Part model, mm, in its own coordinate system. Coordinates: 2 decimals unless noted, no trailing zeros. Write each loop counter-clockwise with the first axis right and the second up, starting at its lowest first coordinate (ties: lowest second). Pieces come first, ordered by that corner, then holes. Notation, with made-up numbers: (51, -5) -> (89, -5) arc R8 cw to (89, -1) -> close; hole circle Ø2 at (79.25, 62.5). An arc over 180 degrees is marked (long way). One line per question, with ' | ' between items. Start each with the question number.
Item 1: Saw through at B-B (x = 228.6). List the corners of the cut face in (y, z) (3 decimals), and give its area (3 significant figures).
Item 2: Probe probe 1 along Z at (x, y) = (228.6, 2); probe 2 along X at (y, z) = (0.7, -63.5); probe 3 along Z at (x, y) = (187, 1.05). List the from-to ranges inside material, lowest first. Write a range as [from, to].
Item 3: Saw through at C-C (z = -8.5). List the corners of the cut face in (x, y) (3 decimals).
Item 4: Pin check, flat tips, straight feed: pin 1 (1 mm diameter, centred on y = 1.5, z = -8, fed in from -X); pin 2 (1.6 mm diameter, centred on y = 1, z = -120.5, fed in from +X); pin 3 (1 mm diameter, centred on x = 63.5, y = 2, fed in from +Z). Stop position of each tip, or through.
Item 5: Saw through at D-D (x = 60.5). List the corners of the cut face in (y, z) (3 decimals).
Item 6: Saw through at A-A (z = -63.5). List the corners of the cut face in (x, y) (3 decimals), and give its area (3 significant figures).
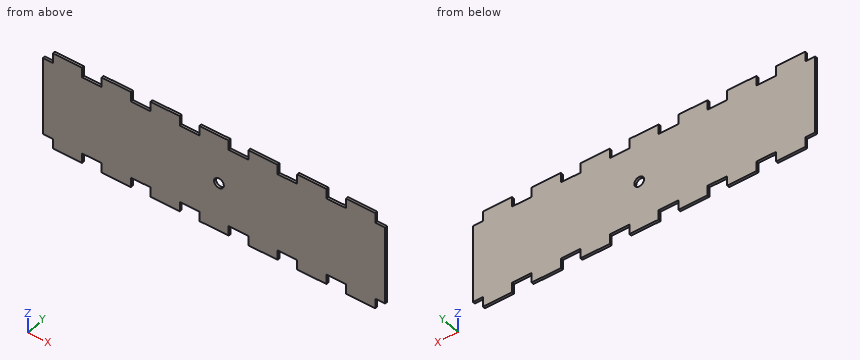
Autodesk Inventor part; units mm, degrees
ref_plane "YZ Plane" through (0, 0, 0) normal (1, 0, 0) x (0, 1, 0)
ref_plane "XZ Plane" through (0, 0, 0) normal (0, 1, 0) x (-1, 0, 0)
ref_plane "XY Plane" through (0, 0, 0) normal (0, 0, 1) x (1, 0, 0)
sketch "Sketch1" plane through (0, 0, 0) normal (0, 1, 0) x (-1, 0, 0)
  line L0 (0, 0) -> (-444.5, 0)
  line L1 (-444.5, 0) -> (-444.5, -127)
  line L2 (-444.5, -127) -> (0, -127)
  line L3 (0, -127) -> (0, 0)
  dimension "d0" = 444.5
  dimension "d1" = 127
extrude "Extrusion1" add sketch "Sketch1" along normal blind 3.175
sketch "Sketch2" plane through (0, 3.175, 0) normal (0, 1, 0) x (1, 0, 0)
  line L0 (0, 127) -> (0, 0)
  line L1 (0, 114.3) -> (12.7, 114.3)
  line L2 (12.7, 114.3) -> (12.7, 127)
  line L3 (444.5, 127) -> (0, 127)
  line L4 (50.8, 127) -> (50.8, 114.3)
  line L5 (50.8, 114.3) -> (76.2, 114.3)
  line L6 (76.2, 114.3) -> (76.2, 127)
  line L7 (114.3, 127) -> (114.3, 114.3)
  line L8 (114.3, 114.3) -> (139.7, 114.3)
  line L9 (139.7, 114.3) -> (139.7, 127)
  line L10 (177.8, 127) -> (177.8, 114.3)
  line L11 (177.8, 114.3) -> (203.2, 114.3)
  line L12 (203.2, 114.3) -> (203.2, 127)
  line L13 (241.3, 127) -> (241.3, 114.3)
  line L14 (241.3, 114.3) -> (266.7, 114.3)
  line L15 (266.7, 114.3) -> (266.7, 127)
  line L16 (304.8, 127) -> (304.8, 114.3)
  line L17 (304.8, 114.3) -> (330.2, 114.3)
  line L18 (330.2, 114.3) -> (330.2, 127)
  line L19 (368.3, 127) -> (368.3, 114.3)
  line L20 (368.3, 114.3) -> (393.7, 114.3)
  line L21 (393.7, 114.3) -> (393.7, 127)
  line L22 (431.8, 127) -> (431.8, 114.3)
  line L23 (431.8, 114.3) -> (444.5, 114.3)
  line L24 (444.5, 0) -> (444.5, 127)
  line L25 (0, 114.3) -> (0, 127)
  line L26 (50.8, 127) -> (76.2, 127)
  line L27 (114.3, 127) -> (139.7, 127)
  line L28 (177.8, 127) -> (203.2, 127)
  line L29 (241.3, 127) -> (266.7, 127)
  line L30 (304.8, 127) -> (330.2, 127)
  line L31 (368.3, 127) -> (393.7, 127)
  line L32 (431.8, 127) -> (444.5, 127)
  line L33 (0, 127) -> (12.7, 127)
  point P0 (444.5, 114.3)
  point P1 (12.7, 127)
  dimension "d4" = 12.7
  dimension "d6" = 12.7
  dimension "d7" = 12.7
  dimension "d8" = 12.7
  dimension "d9" = 25.4
  dimension "d10" = 38.1
  dimension "d11" = 25.4
  dimension "d12" = 38.1
  dimension "d13" = 25.4
  dimension "d14" = 38.1
  dimension "d15" = 25.4
  dimension "d16" = 38.1
  dimension "d17" = 25.4
  dimension "d18" = 38.1
  dimension "d19" = 25.4
  dimension "d20" = 38.1
  dimension "d22" = 0
  dimension "d42" = 12.7
  dimension "d53" = 38.1
extrude "Extrusion2" cut sketch "Sketch2" against normal through all
sketch "Sketch3" plane through (0, 3.175, 0) normal (0, 1, 0) x (1, 0, 0)
  line L0 (0, 0) -> (444.5, 0)
  line L1 (0, 0) -> (12.7, 0)
  line L2 (12.7, 0) -> (12.7, 12.7)
  line L3 (12.7, 12.7) -> (0, 12.7)
  line L4 (0, 12.7) -> (0, 0)
  line L5 (50.8, 0) -> (76.2, 0)
  line L6 (76.2, 0) -> (76.2, 12.7)
  line L7 (76.2, 12.7) -> (50.8, 12.7)
  line L8 (50.8, 12.7) -> (50.8, 0)
  line L9 (114.3, 0) -> (139.7, 0)
  line L10 (139.7, 0) -> (139.7, 12.7)
  line L11 (139.7, 12.7) -> (114.3, 12.7)
  line L12 (114.3, 12.7) -> (114.3, 0)
  line L13 (177.8, 0) -> (203.2, 0)
  line L14 (203.2, 0) -> (203.2, 12.7)
  line L15 (203.2, 12.7) -> (177.8, 12.7)
  line L16 (177.8, 12.7) -> (177.8, 0)
  line L17 (241.3, 0) -> (266.7, 0)
  line L18 (266.7, 0) -> (266.7, 12.7)
  line L19 (266.7, 12.7) -> (241.3, 12.7)
  line L20 (241.3, 12.7) -> (241.3, 0)
  line L21 (304.8, 0) -> (330.2, 0)
  line L22 (330.2, 0) -> (330.2, 12.7)
  line L23 (330.2, 12.7) -> (304.8, 12.7)
  line L24 (304.8, 12.7) -> (304.8, 0)
  line L25 (368.3, 0) -> (393.7, 0)
  line L26 (393.7, 0) -> (393.7, 12.7)
  line L27 (393.7, 12.7) -> (368.3, 12.7)
  line L28 (368.3, 12.7) -> (368.3, 0)
  line L29 (444.5, 0) -> (444.5, 114.3)
  line L30 (444.5, 0) -> (431.8, 0)
  line L31 (431.8, 0) -> (431.8, 12.7)
  line L32 (431.8, 12.7) -> (444.5, 12.7)
  line L33 (444.5, 12.7) -> (444.5, 0)
  point P0 (431.8, 0)
  point P1 (393.7, 0)
  point P2 (330.2, 0)
  point P3 (266.7, 0)
  point P4 (203.2, 0)
  point P5 (139.7, 0)
  point P6 (50.8, 0)
  point P7 (76.2, 0)
  point P8 (12.7, 0)
  dimension "d25" = 12.7
  dimension "d26" = 12.7
  dimension "d27" = 25.4
  dimension "d28" = 38.1
  dimension "d29" = 25.4
  dimension "d30" = 25.4
  dimension "d31" = 25.4
  dimension "d32" = 25.4
  dimension "d33" = 25.4
  dimension "d34" = 12.7
  dimension "d35" = 38.1
  dimension "d36" = 38.1
  dimension "d37" = 38.1
  dimension "d38" = 38.1
  dimension "d39" = 38.1
extrude "Extrusion3" cut sketch "Sketch3" against normal through all
sketch "Sketch4" plane through (0, 3.175, 0) normal (0, 1, 0) x (1, 0, 0)
  circle A0 centre (228.6, 63.5) radius 6.35
  line L0 (0, 114.3) -> (0, 12.7)
  line L1 (241.3, 127) -> (203.2, 127)
  point P0 (0, 0)
  dimension "d43" = 12.7
  dimension "d44" = 228.6
  dimension "d45" = 63.5
hole "Hole1" at (228.6, 3.175, -63.5) direction (0, -1, 0) diameter 12.7 end through all
properties part number "BridgeBottom"
From the geometry:
1) outline: (0, -127) -> (3.175, -127) -> (3.175, -69.85) -> (0, -69.85) -> close; (0, -57.15) -> (3.175, -57.15) -> (3.175, 0) -> (0, 0) -> close | area: 363 mm2
2) probe 1: [-127, -69.85], [-57.15, 0] | probe 2: [0, 222.25], [234.95, 444.5] | probe 3: [-114.3, -12.7]
3) outline: (12.7, 0) -> (50.8, 0) -> (50.8, 3.175) -> (12.7, 3.175) -> close; (76.2, 0) -> (114.3, 0) -> (114.3, 3.175) -> (76.2, 3.175) -> close; (139.7, 0) -> (177.8, 0) -> (177.8, 3.175) -> (139.7, 3.175) -> close; (203.2, 0) -> (241.3, 0) -> (241.3, 3.175) -> (203.2, 3.175) -> close; (266.7, 0) -> (304.8, 0) -> (304.8, 3.175) -> (266.7, 3.175) -> close; (330.2, 0) -> (368.3, 0) -> (368.3, 3.175) -> (330.2, 3.175) -> close; (393.7, 0) -> (431.8, 0) -> (431.8, 3.175) -> (393.7, 3.175) -> close
4) pin 1: x = 12.7 | pin 2: x = 431.8 | pin 3: z = -12.7
5) outline: (0, -114.3) -> (3.175, -114.3) -> (3.175, -12.7) -> (0, -12.7) -> close
6) outline: (0, 0) -> (222.25, 0) -> (222.25, 3.175) -> (0, 3.175) -> close; (234.95, 0) -> (444.5, 0) -> (444.5, 3.175) -> (234.95, 3.175) -> close | area: 1,370 mm2
